Design review of the part built by this model. Coordinates are the model's own, in mm. Face numbers are marked on the shaded views. A direction names the side the tool comes from. Coordinates: 2 decimals unless noted, no trailing zeros. Order: outer loops, then holes, each group sorted by start corner. A loop starts at its lowest first (then second) coordinate and runs counter-clockwise, first axis right, second up. Notation, with made-up numbers: (3, 20) -> (41, 20) arc R25 ccw to (41, 56) -> close; hole circle Ø8 at (72, -10). An arc over 180 degrees is marked (long way). Use a Markdown table: item, result. Add a question column.
Q1. Wall thickness on probe 1 along X at (y, z) = (2.5, -9.25); probe 2 along Z at (x, y) = (18.5, 1); probe 3 along Z at (x, y) = (4.5, 11.1): over which ranges is each line inside the solid? List them lowest first.
Q2. The part is to be moulded in two halves that separate along X. For the marked faces 6, 7, 8 and 9, say which applies: pulls with the +X half, pulls with the -X half, needs draft (parallel to the pull), parting line crosses it, or undercut.
Q3. Insertion check: pin 1 (1.6 mm diameter, centred on x = 5, y = 13, fed in from -Z); pin 2 (4 mm diameter, centred on x = 17.5, z = 4, fed in from +Y); pin 3 (4 mm diameter, centred on x = 24.5, z = -7.55, fed in from -Y); pin 4 (3 mm diameter, centred on x = 4.5, z = 2, fed in from +Y). Each pin has a flat end and moves straight along its axis. Give the tip position at first contact, or say it passes through.
Q4. Add section A-A (z = -1.5). State the section outline as (x, y) points.
Q5. Machinability: for the marked faces 1, 2, 3, 4 and 5, which of the approach directions +Z, -Z, +X, -X, +Y, -Y give a long, thin tool a straight path to every point of the face, cutting with its end or side? Answer none if there is none.
Q6. Add section D-D (x = 4.5). State the section outline as (y, z) points.
Q7. Add section B-B (x = 24.5). State the section outline as (y, z) points, then the cut area to 3 significant figures.
Q8. Add section C-C (y = 5). State the section outline as (x, z) points, then the cut area to 3 significant figures.
from build123d import *

# Parameters (mm, degrees)
SKIZZE2_W                       = 29.5
SKIZZE2_H                       = 15
AUFSATZ_LINEAR_AUSTRAGEN1_DEPTH = 7.5
SKIZZE4_W                       = 27.9
SKIZZE4_H                       = 13.4
SCHNITT_LINEAR_AUSTRAGEN1_DEPTH = 5.7
SKIZZE5_W                       = 29.5
SKIZZE5_H                       = 8.4
AUFSATZ_LINEAR_AUSTRAGEN2_DEPTH = 4
SKIZZE7_W                       = 7.5
SKIZZE7_H                       = 7.2
SKIZZE7_W_2                     = 6.3
SKIZZE7_H_2                     = 6
SKIZZE7_W_3                     = 16.3
SKIZZE7_W_4                     = 15.1
AUFSATZ_LINEAR_AUSTRAGEN3_DEPTH = 2
SKIZZE8_R                       = 1.434086585
SKIZZE8_R_2                     = 1.463442441
SCHNITT_LINEAR_AUSTRAGEN2_DEPTH = 0.5
SKIZZE9_W                       = 10.1
SKIZZE9_H                       = 3
AUFSATZ_LINEAR_AUSTRAGEN4_DEPTH = 6


with BuildPart() as part:
    # Skizze2 → Aufsatz-Linear austragen1 (new body)
    with BuildSketch(Plane(origin=(0, 0, 0), x_dir=(1, 0, 0), z_dir=(0, 1, 0))):
        with Locations((14.75, 7.5)):
            Rectangle(SKIZZE2_W, SKIZZE2_H)
    extrude(amount=AUFSATZ_LINEAR_AUSTRAGEN1_DEPTH)

    # Skizze4 → Schnitt-Linear austragen1 (cut)
    with BuildSketch(Plane.XZ):
        with Locations((14.75, -7.5)):
            Rectangle(SKIZZE4_W, SKIZZE4_H)
    extrude(amount=-SCHNITT_LINEAR_AUSTRAGEN1_DEPTH, mode=Mode.SUBTRACT)

    # Skizze5 → Aufsatz-Linear austragen2 (add)
    with BuildSketch(Plane(origin=(0, 7.5, 0), x_dir=(1, 0, 0), z_dir=(0, 1, 0))):
        with Locations((14.75, 7.55)):
            Rectangle(SKIZZE5_W, SKIZZE5_H)
    extrude(amount=AUFSATZ_LINEAR_AUSTRAGEN2_DEPTH)

    # Skizze7 → Aufsatz-Linear austragen3 (add)
    with BuildSketch(Plane(origin=(0, 11.5, 0), x_dir=(1, 0, 0), z_dir=(0, 1, 0))):
        with Locations((4.5, 7.55)):
            Rectangle(SKIZZE7_W, SKIZZE7_H)
        with Locations((4.5, 7.55)):
            Rectangle(SKIZZE7_W_2, SKIZZE7_H_2, mode=Mode.SUBTRACT)
        with Locations((20.55, 7.55)):
            Rectangle(SKIZZE7_W_3, SKIZZE7_H)
        with Locations((20.55, 7.55)):
            Rectangle(SKIZZE7_W_4, SKIZZE7_H_2, mode=Mode.SUBTRACT)
    extrude(amount=AUFSATZ_LINEAR_AUSTRAGEN3_DEPTH)

    # Skizze8 → Schnitt-Linear austragen2 (cut)
    with BuildSketch(Plane(origin=(0, 11.5, 0), x_dir=(-1, 0, 0), z_dir=(0, 1, 0))):
        with Locations((-4.5, -7.55)):
            Circle(SKIZZE8_R)
        with Locations((-24.5, -7.55)):
            Circle(SKIZZE8_R_2)
    extrude(amount=-SCHNITT_LINEAR_AUSTRAGEN2_DEPTH, mode=Mode.SUBTRACT)

    # Skizze9 → Aufsatz-Linear austragen4 (add)
    with BuildSketch(Plane.XY):
        with Locations((14.75, 4.8)):
            Rectangle(SKIZZE9_W, SKIZZE9_H)
    extrude(amount=AUFSATZ_LINEAR_AUSTRAGEN4_DEPTH)


solid = part.part
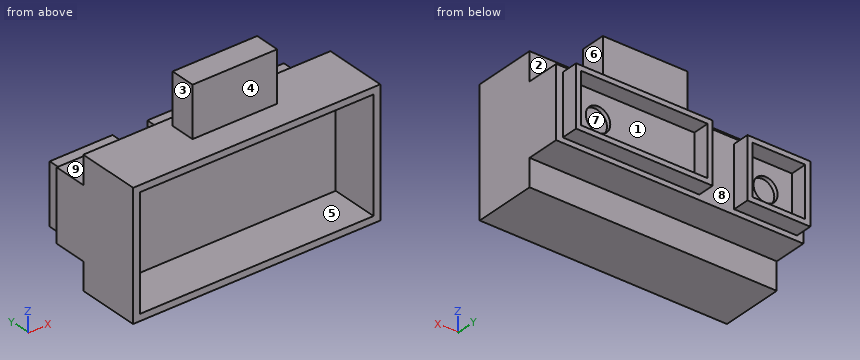
Established:
| question | item | result |
|---|---|---|
| 1 | probe 1 | 0 to 0.8, 28.7 to 29.5 |
| 1 | probe 2 | -15 to -14.2, -0.8 to 0 |
| 1 | probe 3 | -11.75 to -8.98, -6.12 to -3.35 |
| 2 | face 6 | pulls with the +X half |
| 2 | face 7 | undercut |
| 2 | face 8 | undercut |
| 2 | face 9 | needs draft |
| 3 | pin 1 | z = -11.15 |
| 3 | pin 2 | y = 6.3 |
| 3 | pin 3 | y = 5.7 |
| 3 | pin 4 | through |
| 4 | outline | (0, 0) -> (0.8, 0) -> (0.8, 5.7) -> (28.7, 5.7) -> (28.7, 0) -> (29.5, 0) -> (29.5, 7.5) -> (0, 7.5) -> close |
| 5 | face 1 | +Y |
| 5 | face 2 | +Z, +X, -X, +Y |
| 5 | face 3 | +Z, -X, +Y, -Y |
| 5 | face 4 | +Z, +X, -X, -Y |
| 5 | face 5 | -Y |
| 6 | outline | (0, -15) -> (7.5, -15) -> (7.5, -11.75) -> (11.5, -11.75) -> (11.5, -11.15) -> (13.5, -11.15) -> (13.5, -10.55) -> (11.5, -10.55) -> (11.5, -8.98) -> (11, -8.98) -> (11, -6.12) -> (11.5, -6.12) -> (11.5, -4.55) -> (13.5, -4.55) -> (13.5, -3.95) -> (11.5, -3.95) -> (11.5, -3.35) -> (7.5, -3.35) -> (7.5, 0) -> (0, 0) -> (0, -0.8) -> (5.7, -0.8) -> (5.7, -14.2) -> (0, -14.2) -> close |
| 7 | outline | (0, -15) -> (7.5, -15) -> (7.5, -11.75) -> (11.5, -11.75) -> (11.5, -11.15) -> (13.5, -11.15) -> (13.5, -10.55) -> (11.5, -10.55) -> (11.5, -9.01) -> (11, -9.01) -> (11, -6.09) -> (11.5, -6.09) -> (11.5, -4.55) -> (13.5, -4.55) -> (13.5, -3.95) -> (11.5, -3.95) -> (11.5, -3.35) -> (7.5, -3.35) -> (7.5, 0) -> (0, 0) -> (0, -0.8) -> (5.7, -0.8) -> (5.7, -14.2) -> (0, -14.2) -> close |
| 7 | area | 70.7 mm^2 |
| 8 | outline | (0, -15) -> (29.5, -15) -> (29.5, 0) -> (19.8, 0) -> (19.8, 6) -> (9.7, 6) -> (9.7, 0) -> (0, 0) -> close; hole (0.8, -14.2) -> (28.7, -14.2) -> (28.7, -0.8) -> (0.8, -0.8) -> close |
| 8 | area | 129 mm^2 |
